```python
from build123d import *

# Parameters (mm, degrees)
SKETCH2_R                = 80
BOSS_EXTRUDE1_DEPTH      = 6
SKETCH1_R                = 22.5
SKETCH1_R_2              = 3
CUT_EXTRUDE2_DEPTH       = 6
SKETCH3_R                = 30
CUT_EXTRUDE3_DEPTH       = 1
FILLET1_R                = 3
FILLET2_R                = 10
CIRPATTERN1_COUNT        = 2
FILLET1_OF_CIRPATTERN1_R = 3
FILLET2_OF_CIRPATTERN1_R = 10


with BuildPart() as part:
    # Sketch2 → Boss-Extrude1 (new body)
    with BuildSketch(Plane.XY):
        Circle(SKETCH2_R)
    extrude(amount=BOSS_EXTRUDE1_DEPTH)

    # Sketch1 → Cut-Extrude2 (cut)
    with BuildSketch(Plane.XY):
        with Locations((0, 40)):
            Circle(SKETCH1_R)
        with BuildLine():
            ThreePointArc((25.980762112, 24.999999996), (26.699125762, 26.319477951), (27.350531909, 27.673264655))
            Line((27.350531909, 27.673264655), (20.811589784, 31.448524651))
            ThreePointArc((20.811589784, 31.448524651), (19.485571585, 28.75), (17.811589784, 26.252372228))
            Line((17.811589784, 26.252372228), (24.350531909, 22.477112232))
            ThreePointArc((24.350531909, 22.477112232), (25.19724251, 23.718139852), (25.980762112, 24.999999996))
        make_face()
        with BuildLine():
            Line((-20.811589784, 31.448524651), (-27.350531909, 27.673264655))
            ThreePointArc((-27.350531909, 27.673264655), (-26.699125768, 26.319477962), (-25.980762123, 25.000000017))
            ThreePointArc((-25.980762123, 25.000000017), (-25.197242517, 23.718139862), (-24.350531909, 22.477112232))
            Line((-24.350531909, 22.477112232), (-17.811589784, 26.252372228))
            ThreePointArc((-17.811589784, 26.252372228), (-19.485571585, 28.75), (-20.811589784, 31.448524651))
        make_face()
        with BuildLine():
            Line((3, 62.299103121), (3, 69.849623113))
            ThreePointArc((3, 69.849623113), (1.501883253, 69.962382193), (2e-09, 70))
            ThreePointArc((2e-09, 70), (-1.501883251, 69.962382193), (-3, 69.849623113))
            Line((-3, 69.849623113), (-3, 62.299103121))
            ThreePointArc((-3, 62.299103121), (0, 62.5), (3, 62.299103121))
        make_face()
        with BuildLine():
            ThreePointArc((-24.350531909, 22.477112232), (-25.197242517, 23.718139862), (-25.980762123, 25.000000017))
            ThreePointArc((-25.980762123, 25.000000017), (-25.681060849, 24.276457145), (-25.578838325, 23.5))
            ThreePointArc((-25.578838325, 23.5), (-25.980762114, 22), (-27.078838325, 20.901923789))
            Line((-27.078838325, 20.901923789), (-24.350531909, 22.477112232))
        make_face()
        with BuildLine():
            ThreePointArc((-25.980762123, 25.000000017), (-26.699125768, 26.319477962), (-27.350531909, 27.673264655))
            Line((-27.350531909, 27.673264655), (-30.078838325, 26.098076211))
            ThreePointArc((-30.078838325, 26.098076211), (-27.802381199, 26.397777481), (-25.980762123, 25.000000017))
        make_face()
        with Locations((-28.578838325, 23.5)):
            Circle(SKETCH1_R_2)
        with BuildLine():
            Line((30.078838325, 26.098076211), (27.350531909, 27.673264655))
            ThreePointArc((27.350531909, 27.673264655), (26.699125762, 26.319477951), (25.980762112, 24.999999996))
            ThreePointArc((25.980762112, 24.999999996), (27.802381188, 26.397777478), (30.078838325, 26.098076211))
        make_face()
        with BuildLine():
            ThreePointArc((27.078838325, 20.901923789), (25.681060847, 22.723542863), (25.980762112, 24.999999996))
            ThreePointArc((25.980762112, 24.999999996), (25.19724251, 23.718139852), (24.350531909, 22.477112232))
            Line((24.350531909, 22.477112232), (27.078838325, 20.901923789))
        make_face()
        with Locations((28.578838325, 23.5)):
            Circle(SKETCH1_R_2)
        with BuildLine():
            Line((3, 69.849623113), (3, 73))
            ThreePointArc((3, 73), (2.121320344, 70.878679657), (2e-09, 70))
            ThreePointArc((2e-09, 70), (1.501883253, 69.962382193), (3, 69.849623113))
        make_face()
        with Locations((0, 73)):
            Circle(SKETCH1_R_2)
        with BuildLine():
            ThreePointArc((2e-09, 70), (-2.121320343, 70.878679656), (-3, 73))
            Line((-3, 73), (-3, 69.849623113))
            ThreePointArc((-3, 69.849623113), (-1.501883251, 69.962382193), (2e-09, 70))
        make_face()
    cut_extrude2 = extrude(amount=CUT_EXTRUDE2_DEPTH, mode=Mode.SUBTRACT)

    # Sketch3 → Cut-Extrude3 (cut)
    with BuildSketch(Plane.XY.offset(6)):
        with Locations((0, 40)):
            Circle(SKETCH3_R)
    cut_extrude3 = extrude(amount=-CUT_EXTRUDE3_DEPTH, mode=Mode.SUBTRACT)

    # Fillet1
    fillet1_edges = [part.edges().sort_by_distance(p)[0] for p in [
        (24.350531909, 22.477112232, 5.5),
        (27.350531909, 27.673264655, 5.5),
        (3, 69.849623113, 5.5),
        (-3, 69.849623113, 5.5),
        (-27.350531909, 27.673264655, 5.5),
        (-24.350531909, 22.477112232, 5.5),
    ]]
    fillet(fillet1_edges, radius=FILLET1_R)

    # Fillet2
    fillet2_edges = [part.edges().sort_by_distance(p)[0] for p in [
        (17.811589784, 26.252372228, 2.5),
        (-17.811589784, 26.252372228, 2.5),
        (-20.811589784, 31.448524651, 2.5),
        (-3, 62.299103121, 2.5),
        (3, 62.299103121, 2.5),
        (20.811589784, 31.448524651, 2.5),
    ]]
    fillet(fillet2_edges, radius=FILLET2_R)

    # CirPattern1: Cut-Extrude2, Cut-Extrude3 ×2 about axis
    cirpattern1_axis = Axis((0, 0, 0), (0, 0, 1))
    for i in range(1, CIRPATTERN1_COUNT):
        add(cut_extrude2.rotate(cirpattern1_axis, i * 360 / CIRPATTERN1_COUNT), mode=Mode.SUBTRACT)
        add(cut_extrude3.rotate(cirpattern1_axis, i * 360 / CIRPATTERN1_COUNT), mode=Mode.SUBTRACT)

    # Fillet1 of CirPattern1
    fillet1_of_cirpattern1_edges = [part.edges().sort_by_distance(p)[0] for p in [
        (-24.350531909, -22.477112232, 5.5),
        (-27.350531909, -27.673264655, 5.5),
        (-3, -69.849623113, 5.5),
        (3, -69.849623113, 5.5),
        (27.350531909, -27.673264655, 5.5),
        (24.350531909, -22.477112232, 5.5),
    ]]
    fillet(fillet1_of_cirpattern1_edges, radius=FILLET1_OF_CIRPATTERN1_R)

    # Fillet2 of CirPattern1
    fillet2_of_cirpattern1_edges = [part.edges().sort_by_distance(p)[0] for p in [
        (-17.811589784, -26.252372228, 2.5),
        (17.811589784, -26.252372228, 2.5),
        (20.811589784, -31.448524651, 2.5),
        (3, -62.299103121, 2.5),
        (-3, -62.299103121, 2.5),
        (-20.811589784, -31.448524651, 2.5),
    ]]
    fillet(fillet2_of_cirpattern1_edges, radius=FILLET2_OF_CIRPATTERN1_R)


solid = part.part
```
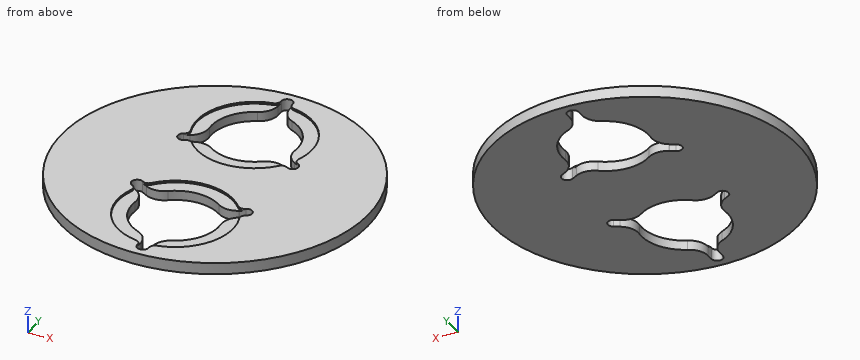
Build history of the part. All positions in model axes, mm. Coordinates: 2 decimals unless noted, no trailing zeros. Order: outer loops, then holes, each group sorted by start corner. A loop starts at its lowest first (then second) coordinate and runs counter-clockwise, first axis right, second up. Notation, with made-up numbers: M -6,88.25 L -2,88.25 A23 cw -2,104.25 Z; hole C -36,62 d4. An arc over 180 degrees is marked long. One line per question, with ' | ' between items. Start each with the question number.
1. Cut at A-A (x = 0). Write the cut outline in (y, z).
2. Cut at C-C (y = -14). Write the cut outline in (x, z), plus the area to 3 significant figures.
3. Cut at B-B (y = -54). Write the cut outline in (x, z), plus the area to 3 significant figures.
4. Cut at D-D (z = 4.1). Count the separate pieces of the cut face and the enclosed holes in it, plus the area to 3 significant figures.
5. Flat gauge pins, fed straight in: P1, Ø1.5, axis at y = 47.5, z = 2, coming from the -X side; P2, Ø1, axis at y = -71, z = 2, coming from the -X side; P3, Ø1.5, axis at y = -56, z = 2, coming from the +X side; P4, Ø2, axis at x = 57.5, y = -44.5, coming from the -Z side. Where does each tip first touch, or does it go through?
6. Wall check: line 1 along Y through (x, z) = (-17, 4.25); line 2 along Y through (x, z) = (30, 4.7); line 3 along X through (y, z) = (46.5, 1.35). Give the ranges that are in metal, low to high. Write a range as [from, to].
The answers:
1) outline: M -80,0 L -76,0 L -76,6 L -80,6 Z; M -17.5,0 L 17.5,0 L 17.5,5 L 10,5 L 10,6 L -10,6 L -10,5 L -17.5,5 Z; M 76,0 L 80,0 L 80,6 L 76,6 Z
2) outline: M -78.77,0 L 78.77,0 L 78.77,6 L 14.97,6 L 14.97,5 L -14.97,5 L -14.97,6 L -78.77,6 Z | area: 915 mm2
3) outline: M -59.03,0 L -17.61,0 L -17.61,5 L -26.53,5 L -26.53,6 L -59.03,6 Z; M 17.61,0 L 59.03,0 L 59.03,6 L 26.53,6 L 26.53,5 L 17.61,5 Z | area: 479 mm2
4) separate pieces: 1 | enclosed holes: 2 | area: 16,300 mm2
5) P1: stops at x = -64.92 | P2: stops at x = -37.81 | P3: stops at x = 57.86 | P4: stops at z = 0
6) line 1: y = [-78.17, -54.74], [-23.58, 23.58], [54.74, 78.17] | line 2: y = [-74.16, -26.14], [-20.86, 20.86], [26.14, 74.16] | line 3: x = [-65.1, -21.54], [21.54, 65.1]
